from build123d import *

# Parameters (mm, degrees)
SKETCH_1_R          = 11
SKETCH_1_R_2        = 1.5
EXTRUDE_1_DEPTH     = 2
SKETCH_4_R          = 5
EXTRUDE_3_DEPTH     = 10
SKETCH_5_R          = 1.5
CUT_EXTRUDE_2_DEPTH = 20.646882704


with BuildPart() as part:
    # 草图1 → 凸台-拉伸1 (new body)
    with BuildSketch(Plane.XY):
        Circle(SKETCH_1_R)
        with Locations((0, 8)):
            Circle(SKETCH_1_R_2, mode=Mode.SUBTRACT)
        with Locations((8, 0)):
            Circle(SKETCH_1_R_2, mode=Mode.SUBTRACT)
        with Locations((0, -8)):
            Circle(SKETCH_1_R_2, mode=Mode.SUBTRACT)
        with Locations((-8, 0)):
            Circle(SKETCH_1_R_2, mode=Mode.SUBTRACT)
    extrude(amount=EXTRUDE_1_DEPTH)

    # 草图4 → 凸台-拉伸3 (add)
    with BuildSketch(Plane.XY.offset(2)):
        Circle(SKETCH_4_R)
    extrude(amount=EXTRUDE_3_DEPTH)

    # 草图5 → 切除-拉伸2 (cut, through all)
    with BuildSketch(Plane.XY.offset(12)):
        Circle(SKETCH_5_R)
    extrude(amount=-CUT_EXTRUDE_2_DEPTH, mode=Mode.SUBTRACT)


solid = part.part
Geometry check sheet. Reference: the model listing, model coordinates, mm. A direction names the side the tool comes from. Coordinates: 2 decimals unless noted, no trailing zeros. Order: outer loops, then holes, each group sorted by start corner. A loop starts at its lowest first (then second) coordinate and runs counter-clockwise, first axis right, second up. Notation, with made-up numbers: (14.5, 40) -> (62.5, 40) arc R30 ccw to (62.5, 72) -> close; hole circle Ø7 at (72, -7). An arc over 180 degrees is marked (long way). Use a Markdown table: item, result. Add a question column.
1. Mould release check, pull along Y, two halves, no side actions. Record for faces 1 (the face through (-1.08, -4.88, 6.93)), 2 (the face through (0, -2, 0)), 3 (the face through (6.5, 0.07, 0.99)): pulls with the +Y half, pulls with the -Y half, needs draft (parallel to the pull), parting line crosses it, or undercut.
2. Cross-section at C-C (x = 8.25). Enter the section's corners in (y, z), and give its area (3 significant figures).
3. Go/stop test with flat-tipped pins: pin 1 Ø3.5 at (x, y) = (8, 0) entering from +Z; pin 2 Ø3 at (x, z) = (-1.5, 10.5) entering from -Y; pin 3 Ø1 at (x, z) = (3.5, 4.5) entering from +Y. Record where each tip stops, or that it passes through.
4. Set-up check for faces 4 (the face through (-1.2, 1.2, 12)), 5 (the face through (5, -2, 2)): record each of +Z, -Z, +X, -X, +Y, -Y from which the full face is reachable in a straight line by a thin tool's end or side.
5. Cross-section at A-A (x = 0). Enter the section's corners in (y, z).
6. Cross-section at D-D (y = 8). Enter the section's corners in (x, z), and give its area (3 significant figures).
7. Material ranges on L1, parallel to Y at x = 0, z = 1.55; L2, parallel to Y at x = 0, z = 6; L3, parallel to Y at x = -0.5, z = 0.75, recorded low to high.
Filled sheet:
| question | item | result |
|---|---|---|
| 1 | face 1 | parting line crosses it |
| 1 | face 2 | needs draft |
| 1 | face 3 | undercut |
| 2 | outline | (-7.28, 0) -> (-1.48, 0) -> (-1.48, 2) -> (-7.28, 2) -> close; (1.48, 0) -> (7.28, 0) -> (7.28, 2) -> (1.48, 2) -> close |
| 2 | area | 23.2 mm2 |
| 3 | pin 1 | z = 2 |
| 3 | pin 2 | y = -5 |
| 3 | pin 3 | y = 4 |
| 4 | face 4 | +Z, +X, -X, +Y, -Y |
| 4 | face 5 | +Z |
| 5 | outline | (-11, 0) -> (-9.5, 0) -> (-9.5, 2) -> (-11, 2) -> close; (-6.5, 0) -> (-1.5, 0) -> (-1.5, 12) -> (-5, 12) -> (-5, 2) -> (-6.5, 2) -> close; (1.5, 0) -> (6.5, 0) -> (6.5, 2) -> (5, 2) -> (5, 12) -> (1.5, 12) -> close; (9.5, 0) -> (11, 0) -> (11, 2) -> (9.5, 2) -> close |
| 6 | outline | (-7.55, 0) -> (-1.5, 0) -> (-1.5, 2) -> (-7.55, 2) -> close; (1.5, 0) -> (7.55, 0) -> (7.55, 2) -> (1.5, 2) -> close |
| 6 | area | 24.2 mm2 |
| 7 | L1 | -11 to -9.5, -6.5 to -1.5, 1.5 to 6.5, 9.5 to 11 |
| 7 | L2 | -5 to -1.5, 1.5 to 5 |
| 7 | L3 | -10.99 to -9.41, -6.59 to -1.41, 1.41 to 6.59, 9.41 to 10.99 |
